Can you work these out from the model? Positions are in its coordinate system, mm. Give positions to 0.01 mm unless a question says otherwise; leave off trailing zeros. Write each loop counter-clockwise with the first axis right and the second up, starting at its lowest first coordinate (ties: lowest second). Pieces come first, ordered by that corner, then holes.
```python
from build123d import *

# Parameters (mm, degrees)
F0_R     = 12.7
F1_ANGLE = 140
F2_DEPTH = 25.4
F3_T     = -2.54


with BuildPart() as f1:
    # F0 (on Top) → F1 (revolve)
    with BuildSketch(Plane.XY):
        Circle(F0_R)
    revolve(axis=Axis((38.1, -3.6203619093, 0), (0, 1, 0)), revolution_arc=F1_ANGLE)

    # F2 (add): a face of the model
    f2_faces = [f1.faces().sort_by_distance(p)[0] for p in [
        (0, 0, 0),
    ]]
    extrude(f2_faces, amount=F2_DEPTH)

    # F3
    f3_openings = [f1.faces().sort_by_distance(p)[0] for p in [
        (0, 0, -25.4),
        (67.286293, 0, 24.490208),
    ]]
    offset(amount=F3_T, openings=f3_openings)


solid = f1.part
```
1) Suppose I cut it at A-A on y = 0. Write out the boundary of the cut face in (x, z), plus the area to 3 significant figures.
Values follow:
outline: (-12.7, -25.4) - (-10.16, -25.4) - (-10.16, 0) arc R48.26 cw to (75.07, 31.02) - (77.02, 32.65) arc R50.8 ccw to (-12.7, 0) - close; (10.16, -25.4) - (12.7, -25.4) - (12.7, 0) arc R25.4 cw to (57.56, 16.33) - (59.5, 17.96) arc R27.94 ccw to (10.16, 0) - close
area: 602 mm2
2) For pin 1 Ø3 at (x, y) = (29, 3.5) entering from -Z; pin 2 Ø4 at (y, z) = (-10, 36.5) entering from +X; pin 3 Ø1 at (y, z) = (3.5, -8.5) entering from +X, each with a flat end and sliding along its axis, tell me the tip position at first contact or that it passes through.
Values follow:
pin 1: stops at z = 23.5
pin 2: stops at x = 70.07
pin 3: stops at x = 12.34
3) Suppose I cut it at B-B on y = 7.5. Write out the boundary of the cut face in (x, z), plus the area to 3 significant figures.
Values follow:
outline: (-10.25, -25.4) - (-6.85, -25.4) - (-6.85, 0) arc R44.95 cw to (72.54, 28.9) - (75.14, 31.08) arc R48.35 ccw to (-10.25, 0) - close; (6.85, -25.4) - (10.25, -25.4) - (10.25, 0) arc R27.85 cw to (59.44, 17.9) - (62.04, 20.08) arc R31.25 ccw to (6.85, 0) - close
area: 805 mm2
4) If we mould it in two halves opening along X, with no side actions, what happens to faces 1 (the face through (-1.323, 10.074, -12.522)), 2 (the face through (67.3, 10.4, 24.5)), 3 (the face through (-2.75, -12.4, -12.52))? For each: +X half, -X half, draft (parallel to the pull), parting line (faces both ways), or undercut.
Values follow:
face 1: undercut
face 2: +X half
face 3: parting line
5) Please list where these lines run through material, in increasing order: L1, parallel to Y at x = 0, z = -10; L2, parallel to Z at x = 58, y = 0.25; L3, parallel to Z at x = 54.5, y = -3.75.
Values follow:
L1: y = -12.7 to -10.16, 10.16 to 12.7
L2: z = 16.7 to 19.62, 43.96 to 46.74
L3: z = 20.13 to 23.5, 44.62 to 47.48
